Geometry check sheet. Reference: the model listing, model coordinates, mm. Face numbers are marked on the shaded views. A direction names the side the tool comes from. Give positions to 0.01 mm unless a question says otherwise; leave off trailing zeros. Write each loop counter-clockwise with the first axis right and the second up, starting at its lowest first coordinate (ties: lowest second). Pieces come first, ordered by that corner, then holes. Notation, with made-up numbers: M 19,70.25 L 50,70.25 A20 cw 50,105.25 Z; hole C -37,16 d11. An arc over 180 degrees is marked long. Write each question's results on one line, items separated by ' | '.
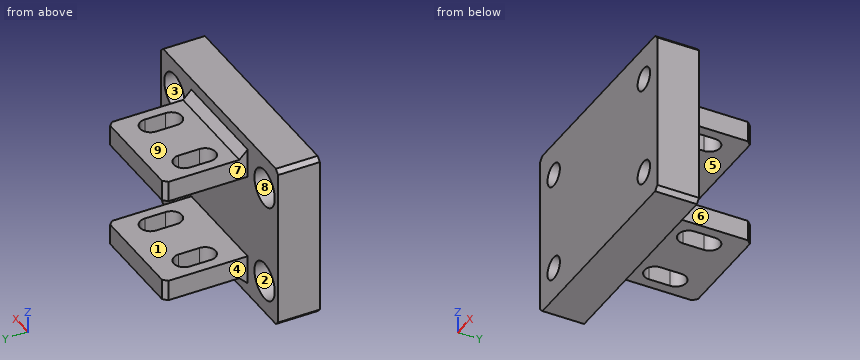
```python
from build123d import *

# Parameters (mm, degrees)
SKETCH1_W           = 52
SKETCH1_H           = 40
SKETCH1_R           = 2.75
BOSS_EXTRUDE1_DEPTH = 10
SKETCH4_R           = 4.5
CUT_EXTRUDE2_DEPTH  = 5
BOSS_EXTRUDE2_START = -13.5
SKETCH2_W           = 5
SKETCH2_H           = 20
BOSS_EXTRUDE2_DEPTH = 25
CUT_EXTRUDE1_REACH  = 55.09
CHAMFER1_SIZE       = 2
CHAMFER2_SIZE       = 1


with BuildPart() as part:
    # Sketch1 → Boss-Extrude1 (new body)
    with BuildSketch(Plane(origin=(0, 0, 0), x_dir=(1, 0, 0), z_dir=(0, 1, 0))):
        Rectangle(SKETCH1_W, SKETCH1_H)
        with Locations(Location((-20, 12, 0), (0, 0, 270))):
            Circle(SKETCH1_R, mode=Mode.SUBTRACT)
        with Locations(Location((20, 12, 0), (0, 0, 270))):
            Circle(SKETCH1_R, mode=Mode.SUBTRACT)
        with Locations(Location((20, -12, 0), (0, 0, 270))):
            Circle(SKETCH1_R, mode=Mode.SUBTRACT)
        with Locations(Location((-20, -12, 0), (0, 0, 270))):
            Circle(SKETCH1_R, mode=Mode.SUBTRACT)
    extrude(amount=BOSS_EXTRUDE1_DEPTH)

    # Sketch4 → Cut-Extrude2 (cut)
    with BuildSketch(Plane(origin=(0, 10, 0), x_dir=(1, 0, 0), z_dir=(0, 1, 0))):
        with Locations(Location((-20, 12, 0), (0, 0, 270))):
            Circle(SKETCH4_R)
        with Locations(Location((20, 12, 0), (0, 0, 270))):
            Circle(SKETCH4_R)
        with Locations(Location((20, -12, 0), (0, 0, 270))):
            Circle(SKETCH4_R)
        with Locations(Location((-20, -12, 0), (0, 0, 270))):
            Circle(SKETCH4_R)
    extrude(amount=-CUT_EXTRUDE2_DEPTH, mode=Mode.SUBTRACT)

    # Sketch2 → Boss-Extrude2 (add)
    with BuildSketch(Plane(origin=(26, 0, 0), x_dir=(0, 0, -1), z_dir=(1, 0, 0)).offset(BOSS_EXTRUDE2_START)):
        with Locations((-12.75, 20)):
            Rectangle(SKETCH2_W, SKETCH2_H)
        with Locations((12.75, 20)):
            Rectangle(SKETCH2_W, SKETCH2_H)
    extrude(amount=-BOSS_EXTRUDE2_DEPTH)

    # Cut-Extrude1: up to this face of the body (flat: up to its plane)
    cut_extrude1_end = Plane(part.part.faces().sort_by_distance((0, 20, -15.25))[0])
    # Sketch3 → Cut-Extrude1 (cut, up to the picked face)
    with BuildSketch(Plane.XY.offset(15.25), mode=Mode.PRIVATE) as cut_extrude1_sk1:
        with BuildLine():
            Line((-5, 22.5), (-5, 17.5))
            ThreePointArc((-5, 17.5), (-7.5, 15), (-10, 17.5))
            Line((-10, 17.5), (-10, 22.5))
            ThreePointArc((-10, 22.5), (-7.5, 25), (-5, 22.5))
        make_face()
    cut_extrude1_tool1 = split(extrude(cut_extrude1_sk1.sketch, amount=-CUT_EXTRUDE1_REACH, mode=Mode.PRIVATE), bisect_by=cut_extrude1_end, keep=Keep.BOTH, mode=Mode.PRIVATE)
    # Sketch3 → Cut-Extrude1 (cut, up to the picked face)
    with BuildSketch(Plane.XY.offset(15.25), mode=Mode.PRIVATE) as cut_extrude1_sk2:
        with BuildLine():
            Line((10, 22.5), (10, 17.5))
            ThreePointArc((10, 17.5), (7.5, 15), (5, 17.5))
            Line((5, 17.5), (5, 22.5))
            ThreePointArc((5, 22.5), (7.5, 25), (10, 22.5))
        make_face()
    cut_extrude1_tool2 = split(extrude(cut_extrude1_sk2.sketch, amount=-CUT_EXTRUDE1_REACH, mode=Mode.PRIVATE), bisect_by=cut_extrude1_end, keep=Keep.BOTH, mode=Mode.PRIVATE)
    add(cut_extrude1_tool1.solids().sort_by(Axis((-7.5, 20, 15.25), (0, 0, -1)))[0], mode=Mode.SUBTRACT)
    add(cut_extrude1_tool2.solids().sort_by(Axis((7.5, 20, 15.25), (0, 0, -1)))[0], mode=Mode.SUBTRACT)

    # Chamfer1
    chamfer1_edges = [part.edges().sort_by_distance(p)[0] for p in [
        (0, 10, 15.25),
        (0, 10, -15.25),
    ]]
    chamfer(chamfer1_edges, length=CHAMFER1_SIZE)

    # Chamfer2
    chamfer2_edges = [part.edges().sort_by_distance(p)[0] for p in [
        (-12.5, 30, 12.75),
        (12.5, 30, 12.75),
        (-12.5, 30, -12.75),
        (12.5, 30, -12.75),
        (26, 5, 20),
        (-26, 5, 20),
        (-26, 5, -20),
        (26, 5, -20),
    ]]
    chamfer(chamfer2_edges, length=CHAMFER2_SIZE)


solid = part.part
```
Q1. Section check A-A (z = -12). State how many separate pieces and enclosed holes the cut face has, then the cut area to 3 significant figures.
Answer key:
separate pieces: 3 | enclosed holes: 2 | area: 785 mm2
Q2. Depth check by flat-ended pin: P1, Ø2.5, axis at x = 21, z = -11, coming from the +Y side; P2, Ø5.5, axis at x = -4, y = 19.5, coming from the +Z side; P3, Ø1.5, axis at y = 20, z = -13, coming from the -X side; P4, Ø5.5, axis at y = 19, z = -14, coming from the +X side. Enter the tip coordinate at first touch or a pass-through.
Answer key:
P1: passes through | P2: stops at z = 15.25 | P3: stops at x = -12.5 | P4: stops at x = 12.5
Q3. Section check C-C (y = 7.75). Enter the section's corners in (x, z), then the cut area to 3 significant figures.
Answer key:
outline: M -26,-19 L -25,-20 L 25,-20 L 26,-19 L 26,19 L 25,20 L -25,20 L -26,19 Z; hole C -20,-12 d9; hole C -20,12 d9; hole C 20,-12 d9; hole C 20,12 d9 | area: 1,820 mm2
Q4. Access from +Z, -Z, +X, -X, +Y, -Y to the whole of each face (thin tool, end or side, straight path). Record for the marked faces 5, 6, 7, 8 and 9.
Answer key:
face 5: +X, -X, +Y | face 6: +Z, -Z, +X, +Y | face 7: +Z, -Z, -X, +Y | face 8: +Y | face 9: +Z, +X, -X, +Y
Q5. Section check D-D (x = 7.5). Enter the section's corners in (y, z), then the cut area to 3 significant figures.
Answer key:
outline: M 0,-20 L 10,-20 L 10,-17.25 L 12,-15.25 L 15,-15.25 L 15,-10.25 L 10,-10.25 L 10,10.25 L 15,10.25 L 15,15.25 L 12,15.25 L 10,17.25 L 10,20 L 0,20 Z; M 25,-15.25 L 30,-15.25 L 30,-10.25 L 25,-10.25 Z; M 25,10.25 L 30,10.25 L 30,15.25 L 25,15.25 Z | area: 504 mm2
Q6. Material ranges on probe 1 along Z at (x, y) = (20, 3.2); probe 2 along X at (y, z) = (7.05, -12); probe 3 along X at (y, z) = (1.7, 12), recorded low to high. Write a range as [from, to].
Answer key:
probe 1: z = [-20, -14.75], [-9.25, 9.25], [14.75, 20] | probe 2: x = [-26, -24.5], [-15.5, 15.5], [24.5, 26] | probe 3: x = [-26, -22.75], [-17.25, 17.25], [22.75, 26]
Q7. Section check B-B (x = 20). Enter the section's corners in (y, z), then the cut area to 3 significant figures.
Answer key:
outline: M 0,-20 L 10,-20 L 10,-16.5 L 5,-16.5 L 5,-14.75 L 0,-14.75 Z; M 0,-9.25 L 5,-9.25 L 5,-7.5 L 10,-7.5 L 10,7.5 L 5,7.5 L 5,9.25 L 0,9.25 Z; M 0,14.75 L 5,14.75 L 5,16.5 L 10,16.5 L 10,20 L 0,20 Z | area: 255 mm2
Q8. Release check for a two-part mould opening along X. For the marked faces 1, 2, 3 and 4 record: released by +X, released by -X, zero draft, split by the parting line, or undercut.
Answer key:
face 1: zero draft | face 2: undercut | face 3: undercut | face 4: released by -X
